```python
from build123d import *

# Parameters (mm, degrees)
SKETCH1_R                            = 3.75
BOSS_EXTRUDE1_DEPTH                  = 15
SKETCH2_W                            = 55
SKETCH2_H                            = 5
BOSS_EXTRUDE2_DEPTH                  = 30
F_3_2_3_2_DIAMETER_HOLE1_D           = 3.2
F_3_2_3_2_DIAMETER_HOLE1_CSINK_D     = 3.25
F_3_2_3_2_DIAMETER_HOLE1_CSINK_ANGLE = 90
CHAMFER1_SIZE                        = 4
FILLET2_R                            = 12.5
CHAMFER2_SIZE                        = 2.5


with BuildPart() as part:
    # Sketch1 → Boss-Extrude1 (new body)
    with BuildSketch(Plane.XY):
        Polygon((0, 0), (-12.5, 0), (-12.5, 92.37), (12.5, 92.37), (12.5, 0), align=None)
        with Locations((0, 82.37)):
            Circle(SKETCH1_R, mode=Mode.SUBTRACT)
    extrude(amount=BOSS_EXTRUDE1_DEPTH)

    # Sketch2 → Boss-Extrude2 (add)
    with BuildSketch(Plane(origin=(0, 0, 0), x_dir=(-1, 0, 0), z_dir=(0, 0, -1))):
        with Locations((0, 2.5)):
            Rectangle(SKETCH2_W, SKETCH2_H)
    extrude(amount=-BOSS_EXTRUDE2_DEPTH)

    # Ø3.2 (3.2) Diameter Hole1 (through all)
    with Locations(Plane(origin=(0, 5, 0), x_dir=(1, 0, 0), z_dir=(0, 1, 0))):
        with Locations((-22.5, -5), (-22.5, -25), (22.5, -25), (22.5, -5)):
            CounterSinkHole(F_3_2_3_2_DIAMETER_HOLE1_D / 2, F_3_2_3_2_DIAMETER_HOLE1_CSINK_D / 2, counter_sink_angle=F_3_2_3_2_DIAMETER_HOLE1_CSINK_ANGLE)

    # Chamfer1
    chamfer1_edges = [part.edges().sort_by_distance(p)[0] for p in [
        (-12.5, 5, 7.5),
        (0, 5, 15),
        (12.5, 5, 7.5),
    ]]
    chamfer(chamfer1_edges, length=CHAMFER1_SIZE)

    # Fillet2
    fillet2_edges = [part.edges().sort_by_distance(p)[0] for p in [
        (12.5, 92.37, 7.5),
        (-12.5, 92.37, 7.5),
    ]]
    fillet(fillet2_edges, radius=FILLET2_R - 0.0001)  # a hair under: the kernel refuses the full size

    # Chamfer2
    chamfer2_edges = [part.edges().sort_by_distance(p)[0] for p in [
        (-3.75, 82.37, 15),
    ]]
    chamfer(chamfer2_edges, length=CHAMFER2_SIZE)


solid = part.part
```
Part model, mm, in its own coordinate system. A direction names the side the tool comes from. Round coordinates to 2 decimals unless told otherwise and drop trailing zeros. Loops run counter-clockwise (first coordinate to the right, second up) from the corner with the lowest first, then second, coordinate; pieces in that order, holes last. Notation, with made-up numbers: (-35, 16) -> (13, 16) arc R14 cw to (13, 21) -> close; hole circle Ø11 at (70, 75). An arc over 180 degrees is marked (long way). Use CSV: the item, a comma, the result in double quotes. Start each with the question number.
1) Wall check: L1, parallel to Z at x = -22.5, y = 1.6; L2, parallel to X at y = 1.4, z = 25; L3, parallel to Y at x = 16.5, z = 24.75. Give the ranges that are in metal, low to high. Write a range as [from, to].
2) Cut at D-D, the plane y = 82.37. Write the cut outline in (x, z), plus the area to 3 significant figures.
3) Cut at C-C, the plane x = 22.5. Write the cut outline in (y, z) (3 decimals).
4) Which spindle directions (+Z, -Z, +X, -X, +Y, -Y) get a long thin tool onto all of the face, cutting with end or side? Do faces 1 (the flat face through (0, 5, 21)), 2 (the flat face through (-27.5, 2, 15)), 3 (the flat face through (-12.5, 44, 7)). Say none if no direction does.
5) Cut at A-A, the plane z = 5. Give the number of separate pieces and of enclosed holes in the cut face, plus the area to 3 significant figures.
6) Cut at B-B, the plane z = 25. Write the cut outline in (x, y) (3 decimals), plus the area to 3 significant figures.
7) Drop flat-ended pins along their axis: P1, Ø3, axis at x = -22.5, z = 5, coming from the -Y side; P2, Ø1.5, axis at x = -7.5, z = 16.5, coming from the +Y side; P3, Ø7.5, axis at x = 5.5, y = 46.5, coming from the +Z side; P4, Ø7.5, axis at y = 51, z = 10.5, coming from the -X side. Give the stop position or say it passes through.
8) Pull direction Z, two halves, no side cores. Call faces 4 (the flat face through (0, 51, 15)), 5 (the cylindrical face through (20.974, 2.453, 4.519)), 6 (the flat face through (12.5, 45, 7)): +Z half, -Z half, draft (parallel to the pull), parting line (faces both ways), or undercut.
Determined:
1,L1,"z = [0, 3.4], [6.6, 23.4], [26.6, 30]"
1,L2,"x = [-27.5, -24.1], [-20.9, 20.9], [24.1, 27.5]"
1,L3,"y = [0, 5]"
2,outline,"(-12.25, 0) -> (-3.75, 0) -> (-3.75, 12.5) -> (-6.25, 15) -> (-12.25, 15) -> close; (3.75, 0) -> (12.25, 0) -> (12.25, 15) -> (6.25, 15) -> (3.75, 12.5) -> close"
2,area,"249 mm2"
3,outline,"(0, 0) -> (5, 0) -> (5, 3.375) -> (4.975, 3.4) -> (0, 3.4) -> close; (0, 6.6) -> (4.975, 6.6) -> (5, 6.625) -> (5, 23.375) -> (4.975, 23.4) -> (0, 23.4) -> close; (0, 26.6) -> (4.975, 26.6) -> (5, 26.625) -> (5, 30) -> (0, 30) -> close"
4,face 1,"+Z, +Y"
4,face 2,"+Z, -Z, -X, +Y, -Y"
4,face 3,"+Z, -Z, -X, +Y"
5,separate pieces,"3"
5,enclosed holes,"1"
5,area,"2,330 mm2"
6,outline,"(-27.5, 0) -> (-24.1, 0) -> (-24.1, 4.975) -> (-24.125, 5) -> (-27.5, 5) -> close; (-20.9, 0) -> (20.9, 0) -> (20.9, 4.975) -> (20.875, 5) -> (-20.875, 5) -> (-20.9, 4.975) -> close; (24.1, 0) -> (27.5, 0) -> (27.5, 5) -> (24.125, 5) -> (24.1, 4.975) -> close"
6,area,"243 mm2"
7,P1,"passes through"
7,P2,"stops at y = 8.25"
7,P3,"stops at z = 15"
7,P4,"stops at x = -12.5"
8,face 4,"+Z half"
8,face 5,"undercut"
8,face 6,"draft"
